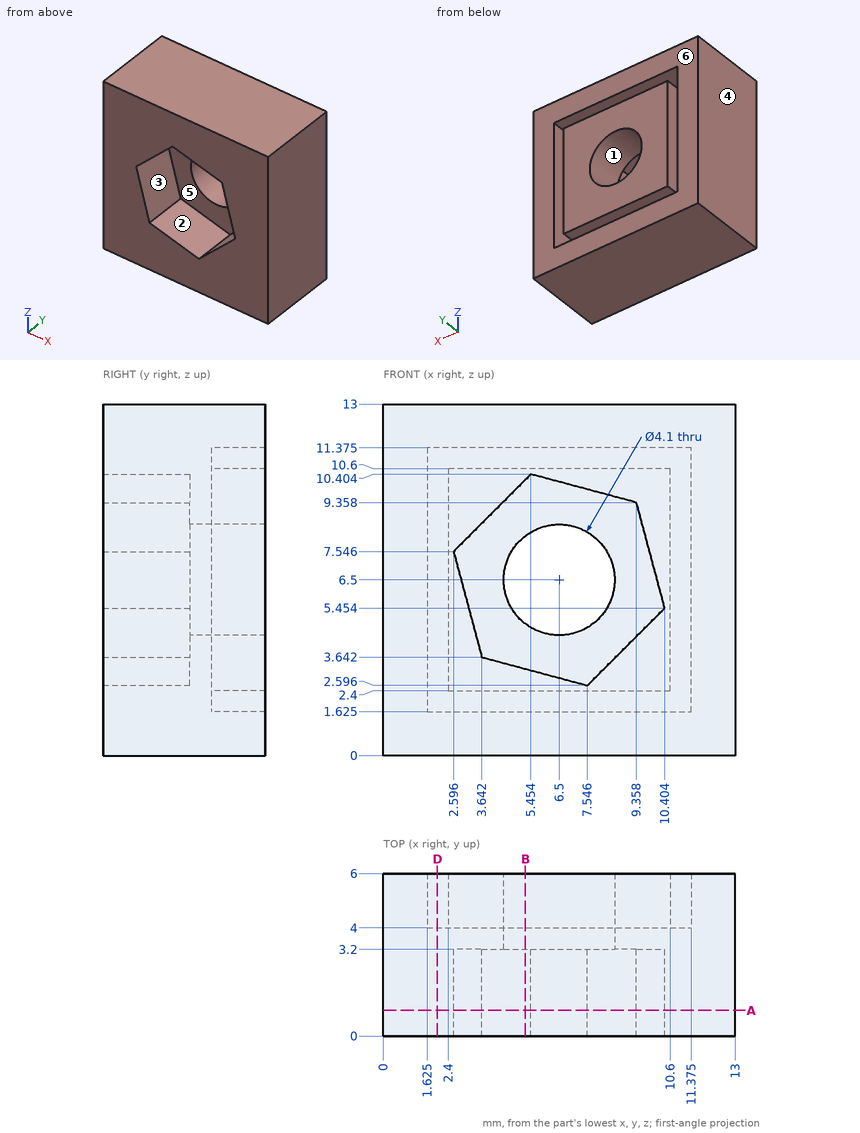
Study the drawing (mm; zero at the part's minimum x, y, z) and answer. A direction names the side the tool comes from. Coordinates: 2 decimals unless noted, no trailing zeros. Write each loop counter-clockwise with the first axis right and the second up, starting at its lowest first coordinate (ties: lowest second). Pieces come first, ordered by that corner, then holes. Notation, with made-up numbers: M -37,-9 L -10,-9 A24 ccw -10,27 Z; hole C 54.5,-14 d8. An arc over 180 degrees is marked long. Use one line per item in the form item = value.
Item 1: Find section A-A, the plane y = 0.95. Give the vertices of the cut face in (x, z), plus the area to 3 significant figures.
Model answer:
outline = M 0,0 L 13,0 L 13,13 L 0,13 Z; hole M 2.6,7.55 L 3.64,3.64 L 7.55,2.6 L 10.4,5.45 L 9.36,9.36 L 5.45,10.4 Z
area = 127 mm2
Item 2: Given P1, Ø6.5, axis at x = 6.5, z = 6.5, coming from the -Y side, flat-ended and moving along its own axis, determine where the tip first touches the part or whether it passes through.
Model answer:
P1 = 3.2
Item 3: The mould has two halves that part along X. Classify the marked faces 3, 4, 5 and 6: released by +X, released by -X, zero draft, split by the parting line, or undercut.
Model answer:
face_3 = undercut
face_4 = released by -X
face_5 = undercut
face_6 = zero draft
Item 4: For the marked faces 1 and 2, determine the directions among +Z, -Z, +X, -X, +Y, -Y from which every point of the face is accessible in a straight line to the end or side of a thin tool.
Model answer:
face_1 = +Y, -Y
face_2 = -Y
Item 5: Find section D-D, the plane x = 2. Give the vertices of the cut face in (y, z) (1 decimal), plus the area to 3 significant figures.
Model answer:
outline = M 0,0 L 6,0 L 6,1.6 L 4,1.6 L 4,11.4 L 6,11.4 L 6,13 L 0,13 Z
area = 58.5 mm2
Item 6: Find section B-B, the plane x = 5.25. Give the vertices of the cut face in (y, z) (1 decimal).
Model answer:
outline = M 0,0 L 6,0 L 6,1.6 L 4,1.6 L 4,2.4 L 6,2.4 L 6,4.9 L 3.2,4.9 L 3.2,3.2 L 0,3.2 Z; M 0,10.2 L 3.2,10.2 L 3.2,8.1 L 6,8.1 L 6,10.6 L 4,10.6 L 4,11.4 L 6,11.4 L 6,13 L 0,13 Z
Item 7: Find the intervals of material crossed by probe 1 along X at (y, z) = (4.6, 9) (1 decimal); probe 2 along Z at (x, y) = (5.25, 4.55) (1 decimal); probe 3 along Z at (x, y) = (6.5, 3.95), in increasing order.
Model answer:
probe_1 = 0 to 1.6, 2.4 to 10.6, 11.4 to 13
probe_2 = 0 to 1.6, 2.4 to 4.9, 8.1 to 10.6, 11.4 to 13
probe_3 = 0 to 4.45, 8.55 to 13
